from build123d import *

# Parameters (mm, degrees)
SKETCH1_R           = 45
SKETCH1_R_2         = 35
BOSS_EXTRUDE1_DEPTH = 2
SKETCH2_R           = 1.75
BOSS_EXTRUDE2_DEPTH = 2
CIRPATTERN1_COUNT   = 16


with BuildPart() as part:
    # Sketch1 → Boss-Extrude1 (new body)
    with BuildSketch(Plane.XY):
        Circle(SKETCH1_R)
        Circle(SKETCH1_R_2, mode=Mode.SUBTRACT)
    extrude(amount=BOSS_EXTRUDE1_DEPTH)

    # Sketch2 → Boss-Extrude2 (add)
    with BuildSketch(Plane.XY):
        with BuildLine():
            ThreePointArc((7.5, 44.370598373), (0, 45), (-7.5, 44.370598373))
            ThreePointArc((-7.5, 44.370598373), (0, 51.870598373), (7.5, 44.370598373))
        make_face()
        with Locations((0, 48)):
            Circle(SKETCH2_R, mode=Mode.SUBTRACT)
    boss_extrude2 = extrude(amount=BOSS_EXTRUDE2_DEPTH)

    # CirPattern1: Boss-Extrude2 ×16 about axis
    cirpattern1_axis = Axis((0, 0, 0), (0, 0, 1))
    for i in range(1, CIRPATTERN1_COUNT):
        add(boss_extrude2.rotate(cirpattern1_axis, i * 360 / CIRPATTERN1_COUNT))


solid = part.part
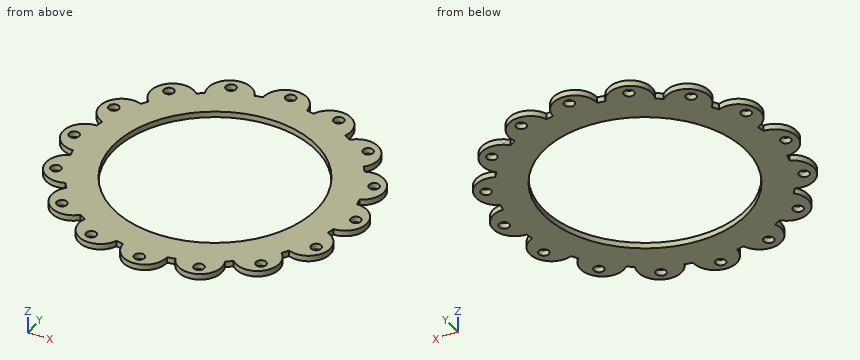
Geometry check sheet. Reference: the model listing, model coordinates, mm. Coordinates: 2 decimals unless noted, no trailing zeros. Loops run counter-clockwise (first coordinate to the right, second up) from the corner with the lowest first, then second, coordinate; pieces in that order, holes last. Notation, with made-up numbers: (88, -23) - (99, -23) arc R23 ccw to (99, 9) - close; hole circle Ø3 at (-0.75, -30.5). An arc over 180 degrees is marked (long way). Use one line per item in the form item = value. Start each with the question number.
Item 1: Thickness scan on probe 1 along Y at (x, z) = (-37, 1.25); probe 2 along Y at (x, z) = (0, 1.65); probe 3 along X at (y, z) = (18.5, 1). Record the ranges inside material, lowest first.
Item 2: Section check C-C, the plane x = 12. Enter the section's corners in (y, z).
Item 3: Gauge pin test, flat ends, axial feed: pin 1 (4 mm diameter, centred on x = 18.37, y = -44.35, fed in from +Z); pin 2 (3 mm diameter, centred on x = -44.35, y = 18.37, fed in from -Z); pin 3 (1 mm diameter, centred on y = 13.5, z = 0.5, fed in from -X). Record the tip position at first contact, or that the pin passes through.
Item 4: Section check D-D, the plane z = 1.65. Give the number of separate pieces and of enclosed holes in the cut face, and give its area (3 significant figures).
Item 5: Section check A-A, the plane x = 0. Enter the section's corners in (y, z), and give its area (3 significant figures).
Item 6: Section check B-B, the plane y = -30.5. Enter the section's corners in (x, z), and give its area (3 significant figures).
Computed:
q1.probe_1 = -36.34 to -26.41, -25.61 to 25.61, 26.41 to 36.34
q1.probe_2 = -51.87 to -49.75, -46.25 to -35, 35 to 46.25, 49.75 to 51.87
q1.probe_3 = -48.34 to -46.09, -42.6 to -29.71, 29.71 to 42.6, 46.09 to 48.34
q2.outline = (-46.6, 0) - (-32.88, 0) - (-32.88, 2) - (-46.6, 2) - close; (32.88, 0) - (46.6, 0) - (46.6, 2) - (32.88, 2) - close
q3.pin_1 = 2
q3.pin_2 = through
q3.pin_3 = -47.88
q4.separate_pieces = 1
q4.enclosed_holes = 17
q4.area = 3,670 mm2
q5.outline = (-51.87, 0) - (-49.75, 0) - (-49.75, 2) - (-51.87, 2) - close; (-46.25, 0) - (-35, 0) - (-35, 2) - (-46.25, 2) - close; (35, 0) - (46.25, 0) - (46.25, 2) - (35, 2) - close; (49.75, 0) - (51.87, 0) - (51.87, 2) - (49.75, 2) - close
q5.area = 53.5 mm2
q6.outline = (-38.82, 0) - (-17.17, 0) - (-17.17, 2) - (-38.82, 2) - close; (17.17, 0) - (38.82, 0) - (38.82, 2) - (17.17, 2) - close
q6.area = 86.6 mm2
